Part model, mm, in its own coordinate system. Face numbers are marked on the shaded views. Coordinates: 2 decimals unless noted, no trailing zeros. Order: outer loops, then holes, each group sorted by start corner. A loop starts at its lowest first (then second) coordinate and runs counter-clockwise, first axis right, second up.
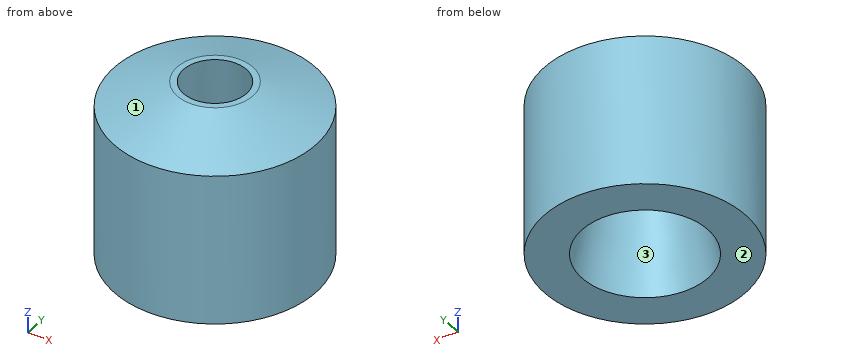
```python
from build123d import *

# Parameters (mm, degrees)
F1_W     = 4
F1_H     = 7
F5_SIZE2 = 2.5
F5_SIZE  = 1


with BuildPart() as f2:
    # F1 (on Right) → F2 (revolve)
    with BuildSketch(Plane.YZ):
        with Locations((2, 3.5)):
            Rectangle(F1_W, F1_H)
    revolve(axis=Axis((0, 0, 3.5), (0, 0, -1)))


with BuildPart() as f3:
    # F0 (on Right) → F3 (revolve)
    with BuildSketch(Plane.YZ):
        Polygon((0, 7), (0, 0), (2.5, 0), (1.25, 7), align=None)
    revolve(axis=Axis((0, 0, 3.5), (0, 0, -1)))


with BuildPart() as f2_1:
    add(f2.part)

    # F4: cut F3
    add(f3.part, mode=Mode.SUBTRACT)

    # F5
    f5_edges = [f2_1.edges().sort_by_distance(p)[0] for p in [
        (0, -4, 7),
    ]]
    f5_side = f2_1.faces().sort_by_distance((0, -4, 3.5))[0]
    chamfer(f5_edges, length=F5_SIZE, length2=F5_SIZE2, reference=f5_side)


solid = f2_1.part
```
(1) Drop flat-ended pins along their axis: pin 1 (4 mm diameter, centred on y = -2, z = 5.5, fed in from -X); pin 2 (1.5 mm diameter, centred on x = -3, z = 2, fed in from +Y). Give the stop position or say it passes through.
(2) Slice it at C-C, the plane z = 5.25. Give the cut face in (x, y) (1 decimal), then the cut area to 3 significant figures.
(3) Slice it at A-A, the plane y = 0. Give the cut face in (x, z), then the cut area to 4 significant figures.
(4) Pull direction X, two halves, no side cores. Call the marked faces 1, 2 and 3: +X half, -X half, draft (parallel to the pull), parting line (faces both ways), or undercut.
(5) Slice it at D-D, the plane z = 3.75. Give the cut face in (x, y), then the cut area to 3 significant figures.
(6) Probe line 1 (X direction, y = -0.5, z = 3.5); line 2 (X direction, y = 1.25, z = 1.5); line 3 (Y direction, x = 2, z = 0.5). List the from-to ranges inside material, lowest first.
Here are the results:
1. pin 1: stops at x = -4
1. pin 2: stops at y = 3.31
2. outline: circle Ø8 at (0, 0); hole circle Ø3.1 at (0, 0)
2. area: 42.6 mm2
3. outline: (-4, 0) - (-2.5, 0) - (-1.25, 7) - (-1.5, 7) - (-4, 6) - close; (1.25, 7) - (2.5, 0) - (4, 0) - (4, 6) - (1.5, 7) - close
3. area: 27.25 mm2
4. face 1: parting line
4. face 2: draft
4. face 3: undercut
5. outline: circle Ø8 at (0, 0); hole circle Ø3.66 at (0, 0)
5. area: 39.7 mm2
6. line 1: x = -3.97 to -1.81, 1.81 to 3.97
6. line 2: x = -3.8 to -1.85, 1.85 to 3.8
6. line 3: y = -3.46 to -1.35, 1.35 to 3.46
